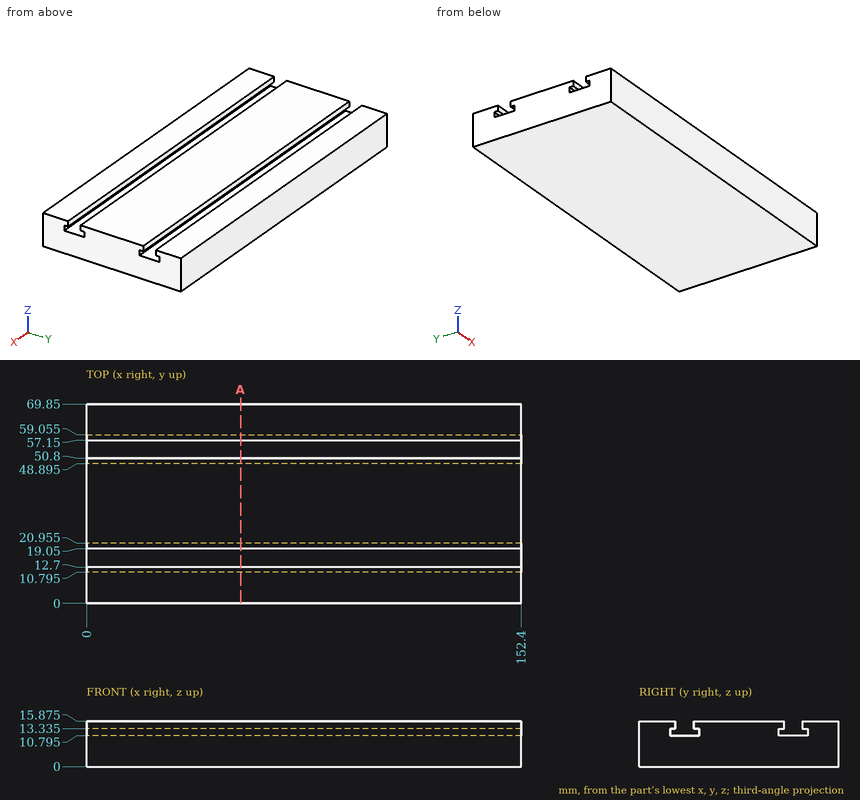
Check sheet for the drawn part. Datum: minimum x, y, z corner. Units: mm. Round coordinates to 2 decimals unless told otherwise and drop trailing zeros. Order: outer loops, then holes, each group sorted by start corner. A loop starts at its lowest first (then second) coordinate and runs counter-clockwise, first axis right, second up. Notation, with made-up numbers: (67.25, -8.75) - (116.25, -8.75) arc R6 ccw to (116.25, -0.75) - close; hole circle Ø10 at (-23, 55.25). An arc over 180 degrees is marked (long way). Use a Markdown table: item, result. Add a question column.
(1) Material ranges on line 1 along Y through (x, z) = (59, 11.5) (3 decimals); line 2 along Y through (x, z) = (94, 13.75); line 3 along Z through (x, y) = (99.5, 56) (3 decimals), recorded low to high. Write a range as [from, to].
(2) Depth check by flat-ended pin: pin 1 (3 mm diameter, centred on x = 74, y = 14.5, fed in from +Z) (3 decimals). Enter the tip coordinate at first touch or a pass-through.
(3) Sectioned sample at A-A, the plane x = 54. Enter the section's corners in (y, z) (3 decimals).
Answers below:
| question | item | result |
|---|---|---|
| 1 | line 1 | [0, 10.795], [20.955, 48.895], [59.055, 69.85] |
| 1 | line 2 | [0, 12.7], [19.05, 50.8], [57.15, 69.85] |
| 1 | line 3 | [0, 10.795] |
| 2 | pin 1 | z = 10.795 |
| 3 | outline | (0, 0) - (69.85, 0) - (69.85, 15.875) - (57.15, 15.875) - (57.15, 13.335) - (59.055, 13.335) - (59.055, 10.795) - (48.895, 10.795) - (48.895, 13.335) - (50.8, 13.335) - (50.8, 15.875) - (19.05, 15.875) - (19.05, 13.335) - (20.955, 13.335) - (20.955, 10.795) - (10.795, 10.795) - (10.795, 13.335) - (12.7, 13.335) - (12.7, 15.875) - (0, 15.875) - close |
